Can you work these out from the model? Positions are in its coordinate system, mm. Give positions to 0.01 mm unless a question says otherwise; leave off trailing zeros. Loops run counter-clockwise (first coordinate to the right, second up) from the corner with the lowest first, then second, coordinate; pieces in that order, holes last. Notation, with made-up numbers: (15, 64.5) -> (19, 64.5) arc R25 cw to (19, 87.5) -> close; hole circle Ø4 at (20.5, 44). An arc over 180 degrees is marked (long way). One line per question, with ' | ' between items.
Autodesk Inventor part; units mm, degrees
ref_plane "Work Plane1" through (14.5, 0, 0) normal (1, 0, 0) x (0, 0, -1)
ref_plane "Work Plane2" through (15, 0, 0) normal (1, 0, 0) x (0, 1, 0)
ref_plane "XZ Plane" through (0, 0, 0) normal (0, 1, 0) x (-1, 0, 0)
sketch "Sketch1" plane through (0, 0, 0) normal (1, 0, 0) x (0, 1, 0)
  circle A0 centre (0, 0) radius 1.25
  dimension "d0" = 2.5
extrude "Extrusion1" add sketch "Sketch1" along normal blind 13
thread "Thread1"
chamfer "Chamfer1" distance 1.25 distance2 2.5 1 edges at (0, -1.25, 0) measured on face at (0, -0.1478, -0.3896)
ref_plane "Work Plane1" through (14.5, 0, 0) normal (1, 0, 0) x (0, 0, -1)
sketch "Sketch2" plane through (14.5, 0, 0) normal (1, 0, 0) x (0, 0, -1)
  circle A0 centre (0, 0) radius 2.5
  dimension "d11" = 5
loft "Loft1" add profiles "Sketch2" section 1 edges at (13, -1.25, 0)
sketch "Sketch3" plane through (0, 0, 0) normal (0, 1, 0) x (-1, 0, 0)
  line L0 (-14.5, -2.5) -> (-14.5, 2.5) construction
  line L1 (-14.5, 0) -> (-15, 0)
  arc A0 (-14.5, 2.5) -> (-15, 0) centre (-8.5, 0) ccw
  line L2 (-14.5, 2.5) -> (-14.5, 0)
  line L3 (3.0248, 0) -> (-18.1485, 0)
  point P0 (0, 0)
  dimension "d16" = 0.5
revolve "Revolution1" add sketch "Sketch3" angle 360 about axis through (-10, 0, 0) along (1, 0, 0)
ref_plane "Work Plane2" through (15, 0, 0) normal (1, 0, 0) x (0, 1, 0)
sketch "Sketch4" plane through (15, 0, 0) normal (1, 0, 0) x (0, 1, 0)
  line L0 (1.25, 0.5) -> (1.25, -0.5)
  line L1 (-1.25, -0.5) -> (-1.25, 0.5)
  line L2 (0.5, -1.25) -> (-0.5, -1.25)
  line L3 (-0.5, 1.25) -> (0.5, 1.25)
  line L4 (-0.5, -1.25) -> (-0.5, -0.5)
  line L5 (-0.5, 0.5) -> (-0.5, 1.25)
  line L6 (1.25, -0.5) -> (0.5, -0.5)
  line L7 (-0.5, -0.5) -> (-1.25, -0.5)
  line L8 (0.5, 1.25) -> (0.5, 0.5)
  line L9 (0.5, -0.5) -> (0.5, -1.25)
  line L10 (-1.25, 0.5) -> (-0.5, 0.5)
  line L11 (0.5, 0.5) -> (1.25, 0.5)
  dimension "d18" = 2.5
  dimension "d19" = 1
  dimension "d20" = 1
  dimension "d21" = 2.5
extrude "Extrusion2" cut sketch "Sketch4" against normal blind 1 draft -10
properties part number "Parafuso do Plug P10"
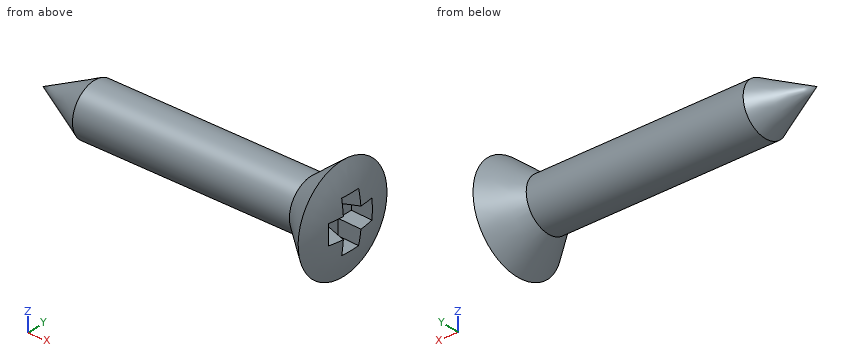
Q1. If I drill on probe 1 along Z at (x, y) = (6.75, 0.25); probe 2 along X at (y, z) = (-1.55, -0.55); probe 3 along Y at (x, z) = (11.5, 1.05), over which ranges is the centre line in solid material (lowest first)? Write a range as from..to.
Entries:
probe 1: -1.22..1.22 | probe 2: 13.47..14.79 | probe 3: -0.68..0.68
Q2. For pin 1 Ø3 at (y, z) = (-2, 1.5) entering from +X; pin 2 Ø1.5 at (y, z) = (-1, 1) entering from -X; pin 3 Ø3 at (x, y) = (7.5, 1) entering from -Z, each with a flat end and sliding along its axis, tell me the tip position at first contact or that it passes through.
Entries:
pin 1: x = 14.92 | pin 2: x = 1.33 | pin 3: z = -1.25
Q3. If we section it at B-B (x = 1.25): Write out the boundary of the cut face in (y, z) (3 decimals), plus the area to 3 significant figures.
Entries:
outline: circle Ø1.25 at (0, 0) | area: 1.23 mm²
Q4. If we section it at A-A (x = 7.25): Write out the boundary of the cut face in (y, z), plus the area to 3 significant figures.
Entries:
outline: circle Ø2.5 at (0, 0) | area: 4.91 mm²
